Autodesk Inventor part; units mm, degrees
ref_plane "YZ Plane" through (0, 0, 0) normal (1, 0, 0) x (0, 1, 0)
ref_plane "XZ Plane" through (0, 0, 0) normal (0, 1, 0) x (-1, 0, 0)
ref_plane "XY Plane" through (0, 0, 0) normal (0, 0, 1) x (1, 0, 0)
sketch "Sketch1" plane through (0, 0, 0) normal (0, 0, 1) x (1, 0, 0)
  line L0 (-10, 11) -> (10, 11)
  line L1 (15, 6) -> (15, -6)
  line L2 (10, -11) -> (-10, -11)
  line L3 (-15, -6) -> (-15, 6)
  line L4 (-15, 11) -> (15, -11) construction
  line L5 (15, 11) -> (-15, -11) construction
  arc A0 (-10, 11) -> (-15, 6) centre (-10, 6) ccw
  arc A1 (15, 6) -> (10, 11) centre (10, 6) ccw
  arc A2 (10, -11) -> (15, -6) centre (10, -6) ccw
  arc A3 (-15, -6) -> (-10, -11) centre (-10, -6) ccw
  point P0 (0, 0)
  dimension "d0" = 22
  dimension "d1" = 30
  dimension "d2" = 5
extrude "Extrusion1" add sketch "Sketch1" along normal blind 6
sketch "Sketch2" plane through (0, 0, 6) normal (0, 0, 1) x (1, 0, 0)
  arc A0 (-10, 11) -> (-15, 6) centre (-10, 6) ccw
  line L0 (-12.5725, 10.2875) -> (-22.5725, 4.2875)
  arc A1 (-22.5725, 4.2875) -> (-22.5725, -4.2875) centre (-20, 0) ccw
  line L1 (-22.5725, -4.2875) -> (-12.5725, -10.2875)
  arc A2 (-15, -6) -> (-10, -11) centre (-10, -6) ccw
  line L2 (-15, 6) -> (-15, -6)
  line L3 (0, 0) -> (0, 5.4971)
  arc A3 (15, 6) -> (10, 11) centre (10, 6) ccw
  line L4 (12.5725, 10.2875) -> (22.5725, 4.2875)
  arc A4 (22.5725, -4.2875) -> (22.5725, 4.2875) centre (20, 0) ccw
  line L5 (22.5725, -4.2875) -> (12.5725, -10.2875)
  arc A5 (10, -11) -> (15, -6) centre (10, -6) ccw
  line L6 (15, 6) -> (15, -6)
  dimension "d5" = 5
  dimension "d6" = 40
extrude "Extrusion2" add sketch "Sketch2" against normal blind 3
sketch "Sketch3" plane through (0, 0, 6) normal (0, 0, 1) x (1, 0, 0)
  circle A0 centre (-20, 0) radius 3
  circle A1 centre (20, 0) radius 3
  arc A2 (-22.5725, 4.2875) -> (-22.5725, -4.2875) centre (-20, 0) ccw
  arc A3 (22.5725, -4.2875) -> (22.5725, 4.2875) centre (20, 0) ccw
  point P0 (0, 0)
  dimension "d9" = 6
  dimension "d10" = 6
extrude "Extrusion3" cut sketch "Sketch3" against normal blind 3
sketch "Sketch4" plane through (0, 0, 6) normal (0, 0, 1) x (1, 0, 0)
  line L0 (-10.15, -11.15) -> (10.15, -11.15)
  line L1 (15.15, -6.15) -> (15.15, 6.15)
  line L2 (10.15, 11.15) -> (-10.15, 11.15)
  line L3 (-15.15, 6.15) -> (-15.15, -6.15)
  line L4 (-15.15, -11.15) -> (15.15, 11.15) construction
  line L5 (15.15, -11.15) -> (-15.15, 11.15) construction
  arc A0 (-10.15, 11.15) -> (-15.15, 6.15) centre (-10.15, 6.15) ccw
  arc A1 (15.15, 6.15) -> (10.15, 11.15) centre (10.15, 6.15) ccw
  arc A2 (10.15, -11.15) -> (15.15, -6.15) centre (10.15, -6.15) ccw
  arc A3 (-15.15, -6.15) -> (-10.15, -11.15) centre (-10.15, -6.15) ccw
  point P0 (0, 0)
  dimension "d13" = 22.3
  dimension "d14" = 30.3
  dimension "d15" = 5
extrude "Extrusion4" add sketch "Sketch4" along normal blind 14
sketch "Sketch5" plane through (0, 0, 0) normal (0, 0, -1) x (-1, 0, 0)
  line L0 (-7, 8) -> (7, 8)
  line L1 (12, 3) -> (12, -4)
  line L2 (8, -8) -> (-8, -8)
  line L3 (-12, -4) -> (-12, 3)
  line L4 (-12, 8) -> (12, -8) construction
  line L5 (12, 8) -> (-12, -8) construction
  line L6 (-12, 3) -> (-7, 8)
  line L7 (7, 8) -> (12, 3)
  arc A0 (-12, -4) -> (-8, -8) centre (-8, -4) ccw
  arc A1 (8, -8) -> (12, -4) centre (8, -4) ccw
  point P0 (0, 0)
  dimension "d18" = 16
  dimension "d19" = 24
  dimension "d20" = 5
  dimension "d21" = 5
  dimension "d22" = 5
  dimension "d23" = 5
  dimension "d24" = 4
extrude "Extrusion5" cut sketch "Sketch5" against normal blind 17
sketch "Sketch7" plane through (0, 0, 17) normal (0, 0, -1) x (-1, 0, 0)
  line L0 (0.5, 3.8693) -> (-0.5, 3.8693)
  line L1 (-0.5, 3.8693) -> (-0.5, 0.6693)
  line L2 (-0.5, 0.6693) -> (0.5, 0.6693)
  line L3 (0.5, 0.6693) -> (0.5, 3.8693)
  line L4 (0.5, 3.8693) -> (-0.5, 0.6693) construction
  line L5 (-0.5, 3.8693) -> (0.5, 0.6693) construction
  line L6 (3.4545, 0.6693) -> (2.4545, 0.6693)
  line L7 (2.4545, 0.6693) -> (2.4545, -2.5307)
  line L8 (2.4545, -2.5307) -> (3.4545, -2.5307)
  line L9 (3.4545, -2.5307) -> (3.4545, 0.6693)
  line L10 (3.4545, 0.6693) -> (2.4545, -2.5307) construction
  line L11 (2.4545, 0.6693) -> (3.4545, -2.5307) construction
  line L12 (0, 0) -> (0, -2.165)
  line L13 (-3.4545, 0.6693) -> (-2.4545, 0.6693)
  line L14 (-2.4545, 0.6693) -> (-2.4545, -2.5307)
  line L15 (-2.4545, -2.5307) -> (-3.4545, -2.5307)
  line L16 (-3.4545, -2.5307) -> (-3.4545, 0.6693)
  line L17 (-3.4545, 0.6693) -> (-2.4545, -2.5307) construction
  line L18 (-2.4545, 0.6693) -> (-3.4545, -2.5307) construction
  point P0 (0, 2.2693)
  point P1 (2.9545, -0.9307)
  point P2 (-2.9545, -0.9307)
  point P3 (-2.9545, 0.6693)
  dimension "d27" = 1
  dimension "d28" = 1
  dimension "d29" = 3.2
  dimension "d30" = 3.2
  dimension "d31" = 0
extrude "Extrusion6" add sketch "Sketch7" along normal blind 14
equation "\"d21\" = d20"
equation "\"d22\" = d20"
equation "\"d23\" = d22"
properties part number "power_socket_24V"
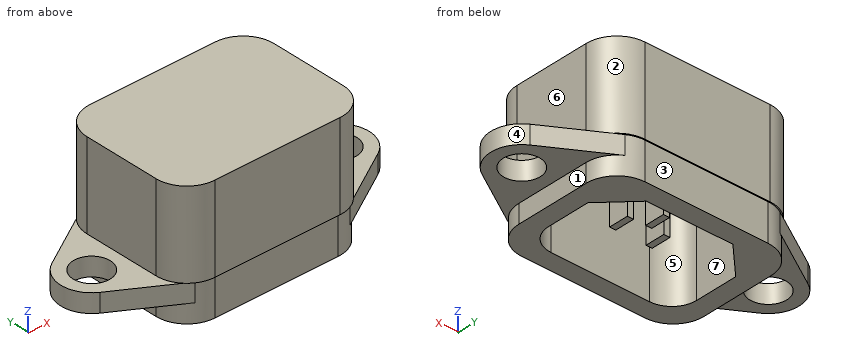
Design review of the part built by this model. Coordinates are the model's own, in mm. Face numbers are marked on the shaded views. A direction names the side the tool comes from. Round coordinates to 2 decimals unless told otherwise and drop trailing zeros. Write each loop counter-clockwise with the first axis right and the second up, starting at its lowest first coordinate (ties: lowest second). Pieces come first, ordered by that corner, then holes. Notation, with made-up numbers: (-26.5, -29) -> (9.5, -29) arc R34 cw to (9.5, 8) -> close; hole circle Ø7 at (36, -29). An arc over 180 degrees is marked (long way). Write item = value, one per line. Start each with the question number.
1) Tool access review of the marked faces 1, 2 and 3: name each direction out of +Z, -Z, +X, -X, +Y, -Y from which nothing blocks a thin tool from reaching the whole face with its end or side.
2) Clearance check with flat-ended pins moving along their axes: pin 1 (5 mm diameter, centred on x = -5.5, y = 2, fed in from -Z); pin 2 (1.8 mm diameter, centred on x = -0.5, z = 2, fed in from +Y); pin 3 (3.5 mm diameter, centred on y = -0.5, z = 13.5, fed in from -X); pin 4 (1.5 mm diameter, centred on x = 18, y = 0.5, fed in from -Z). State where each tip first meets the part, or that it passes through.
3) Take a section at A-A, the plane y = 0. Count the separate pieces of the cut face and the enclosed holes in it, plus the area to 3 significant figures.
4) Take a section at B-B, the plane z = 13.75. State the section outline as (x, y) points.
5) Take a section at D-D, the plane x = 20. State the section outline as (y, z) points.
6) Wall thickness on probe 1 along X at (y, z) = (-0.75, 12); probe 2 along X at (y, z) = (2, 12.25); probe 3 along X at (y, z) = (2.25, 2.75): over which ranges is each line inside the solid? List them lowest first. Write a range as from..to.
7) Mouldability with a two-part tool opening along Y and no side actions: class the marked faces 4, 5, 6 and 7 as +Y half, -Y half, draft (parallel to the pull), parting line (faces both ways), or undercut.
8) Take a section at C-C, the plane z = 2. State the section outline as (x, y) points.
Results list:
q1.face_1 = -Z, +X, +Y, -Y
q1.face_2 = +Z, +X, +Y
q1.face_3 = -Z, +X, -X, +Y
q2.pin_1 = 3
q2.pin_2 = 11
q2.pin_3 = -15.15
q2.pin_4 = through
q3.separate_pieces = 3
q3.enclosed_holes = 0
q3.area = 248 mm²
q4.outline = (-15.15, -6.15) arc R5 ccw to (-10.15, -11.15) -> (10.15, -11.15) arc R5 ccw to (15.15, -6.15) -> (15.15, 6.15) arc R5 ccw to (10.15, 11.15) -> (-10.15, 11.15) arc R5 ccw to (-15.15, 6.15) -> close; (-3.45, -2.53) -> (-2.45, -2.53) -> (-2.45, 0.67) -> (-3.45, 0.67) -> close; (-0.5, 0.67) -> (0.5, 0.67) -> (0.5, 3.87) -> (-0.5, 3.87) -> close; (2.45, -2.53) -> (3.45, -2.53) -> (3.45, 0.67) -> (2.45, 0.67) -> close; hole (-12, -4) arc R4 ccw to (-8, -8) -> (8, -8) arc R4 ccw to (12, -4) -> (12, 3) -> (7, 8) -> (-7, 8) -> (-12, 3) -> close
q5.outline = (-5.83, 3) -> (-3, 3) -> (-3, 6) -> (-5.83, 6) -> close; (3, 3) -> (5.83, 3) -> (5.83, 6) -> (3, 6) -> close
q6.probe_1 = -15.15..-12, -3.45..-2.45, 2.45..3.45, 12..15.15
q6.probe_2 = -15.15..-12, -0.5..0.5, 12..15.15
q6.probe_3 = -15..-12, 12..15
q7.face_4 = parting line
q7.face_5 = undercut
q7.face_6 = draft
q7.face_7 = undercut
q8.outline = (-15, -6) arc R5 ccw to (-10, -11) -> (10, -11) arc R5 ccw to (15, -6) -> (15, 6) arc R5 ccw to (10, 11) -> (-10, 11) arc R5 ccw to (-15, 6) -> close; hole (-12, -4) arc R4 ccw to (-8, -8) -> (8, -8) arc R4 ccw to (12, -4) -> (12, 3) -> (7, 8) -> (-7, 8) -> (-12, 3) -> close
